Build history of the part. All positions in model axes, mm. Round coordinates to 2 decimals unless told otherwise and drop trailing zeros. Order: outer loops, then holes, each group sorted by start corner. A loop starts at its lowest first (then second) coordinate and runs counter-clockwise, first axis right, second up. Notation, with made-up numbers: M -14.5,37.5 L -6.5,37.5 A9 ccw -6.5,46.5 Z; hole C 28,59.25 d5. An arc over 180 degrees is marked long. One line per item, written item: value. Start each with the question number.
Item 1: Probe L1, parallel to Y at x = -13.75, z = 2; L2, parallel to Y at x = 15.75, z = 1.4; L3, parallel to Y at x = 92.25, z = 2.15. List the from-to ranges inside material, lowest first.
Item 2: Band-saw the part on C-C, the plane y = 0. Write the cut outline in (x, z).
Item 3: Band-saw the part on A-A, the plane x = 92.25. Write the cut outline in (y, z).
Item 4: Pin check, flat tips, straight feed: pin 1 (1.9 mm diameter, centred on x = -13.75, y = -13.5, fed in from +Z); pin 2 (1.5 mm diameter, centred on y = 1.5, z = 2, fed in from -X). Stop position of each tip, or through.
Item 5: Band-saw the part on B-B, the plane z = 0.7. Give the number of separate pieces and of enclosed holes in the cut face, then the cut area to 3 significant figures.
```python
from build123d import *

# Parameters (mm, degrees)
BOSS_EXTRUDE1_DEPTH        = 3
M2_CLEARANCE_HOLE1_D       = 2.4
F_3_5_3_5_DIAMETER_HOLE1_D = 3.5


with BuildPart() as part:
    # Sketch1 → Boss-Extrude1 (new body)
    with BuildSketch(Plane.XY):
        Polygon((-17.75, 16), (182.25, 16), (182.25, -16), (-17.75, -16), (-17.75, -10), (12.25, -10), (12.25, 10), (-17.75, 10), align=None)
    extrude(amount=BOSS_EXTRUDE1_DEPTH)

    # M2 Clearance Hole1 (through all)
    with Locations(Plane.XY.offset(3)):
        with Locations((-13.75, 13.5), (-5.75, 13.5), (2.25, 13.5), (10.25, 13.5), (15.75, 8), (15.75, -8), (10.25, -13.5), (2.25, -13.5), (-5.75, -13.5), (-13.75, -13.5)):
            Hole(M2_CLEARANCE_HOLE1_D / 2)

    # Ø3.5 (3.5) Diameter Hole1 (through all)
    with Locations(Plane.XY.offset(3)):
        with Locations((92.25, -9), (92.25, 10), (172.25, 9), (172.25, -9)):
            Hole(F_3_5_3_5_DIAMETER_HOLE1_D / 2)


solid = part.part
```
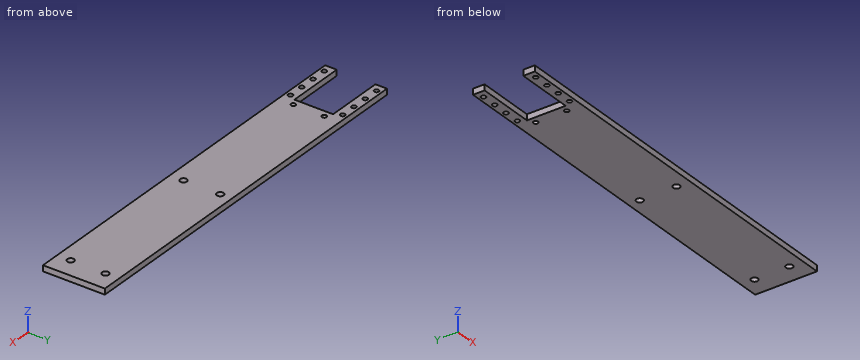
Output:
1. L1: y = -16 to -14.7, -12.3 to -10, 10 to 12.3, 14.7 to 16
1. L2: y = -16 to -9.2, -6.8 to 6.8, 9.2 to 16
1. L3: y = -16 to -10.75, -7.25 to 8.25, 11.75 to 16
2. outline: M 12.25,0 L 182.25,0 L 182.25,3 L 12.25,3 Z
3. outline: M -16,0 L -10.75,0 L -10.75,3 L -16,3 Z; M -7.25,0 L 8.25,0 L 8.25,3 L -7.25,3 Z; M 11.75,0 L 16,0 L 16,3 L 11.75,3 Z
4. pin 1: passes through
4. pin 2: stops at x = 12.25
5. separate pieces: 1
5. enclosed holes: 14
5. area: 5,720 mm²
